```python
from build123d import *

# Parameters (mm, degrees)
SKETCH_2_W          = 100
SKETCH_2_H          = 70
EXTRUDE_1_DEPTH     = 80
SKETCH_4_W          = 96
SKETCH_4_H          = 66
CUT_EXTRUDE_1_DEPTH = 78
FILLET_2_R          = 2.5
SKETCH_6_R          = 5
SKETCH_6_R_2        = 2.3
EXTRUDE_3_DEPTH     = 10


with BuildPart() as part:
    # Эскиз2 → Бобышка-Вытянуть1 (new body)
    with BuildSketch(Plane(origin=(0, 0, 0), x_dir=(1, 0, 0), z_dir=(0, 1, 0))):
        Rectangle(SKETCH_2_W, SKETCH_2_H)
    extrude(amount=EXTRUDE_1_DEPTH)

    # Эскиз4 → Вырез-Вытянуть1 (cut)
    with BuildSketch(Plane(origin=(0, 80, 0), x_dir=(1, 0, 0), z_dir=(0, 1, 0))):
        Rectangle(SKETCH_4_W, SKETCH_4_H)
    extrude(amount=-CUT_EXTRUDE_1_DEPTH, mode=Mode.SUBTRACT)

    # Скругление2
    fillet_2_edges = [part.edges().sort_by_distance(p)[0] for p in [
        (-48, 2, 0),
        (-48, 41, 33),
        (0, 2, -33),
        (-48, 41, -33),
        (48, 2, 0),
        (48, 41, -33),
        (0, 2, 33),
        (48, 41, 33),
        (0, 0, 35),
        (-50, 0, 0),
        (0, 0, -35),
        (50, 0, 0),
        (50, 40, 35),
        (-50, 40, 35),
        (-50, 40, -35),
        (50, 40, -35),
    ]]
    fillet(fillet_2_edges, radius=FILLET_2_R)

    # Эскиз6 → Бобышка-Вытянуть3 (add)
    # profile 1 of 4: a face of its own
    with BuildSketch(Plane(origin=(0, 2, 0), x_dir=(1, 0, 0), z_dir=(0, 1, 0))):
        with Locations(Location((-37.5, 13.725, 0), (0, 0, 270))):
            Circle(SKETCH_6_R)
        with Locations(Location((-37.5, 13.725, 0), (0, 0, 270))):
            Circle(SKETCH_6_R_2, mode=Mode.SUBTRACT)
    # profile 2 of 4: a face of its own
    with BuildSketch(Plane(origin=(0, 2, 0), x_dir=(1, 0, 0), z_dir=(0, 1, 0))):
        with Locations(Location((37.5, 13.725, 0), (0, 0, 270))):
            Circle(SKETCH_6_R)
        with Locations(Location((37.5, 13.725, 0), (0, 0, 270))):
            Circle(SKETCH_6_R_2, mode=Mode.SUBTRACT)
    # profile 3 of 4: a face of its own
    with BuildSketch(Plane(origin=(0, 2, 0), x_dir=(1, 0, 0), z_dir=(0, 1, 0))):
        with Locations(Location((-37.5, -13.725, 0), (0, 0, 270))):
            Circle(SKETCH_6_R)
        with Locations(Location((-37.5, -13.725, 0), (0, 0, 270))):
            Circle(SKETCH_6_R_2, mode=Mode.SUBTRACT)
    # profile 4 of 4: a face of its own
    with BuildSketch(Plane(origin=(0, 2, 0), x_dir=(1, 0, 0), z_dir=(0, 1, 0))):
        with Locations(Location((37.5, -13.725, 0), (0, 0, 270))):
            Circle(SKETCH_6_R)
        with Locations(Location((37.5, -13.725, 0), (0, 0, 270))):
            Circle(SKETCH_6_R_2, mode=Mode.SUBTRACT)
    extrude(amount=EXTRUDE_3_DEPTH)


solid = part.part
```
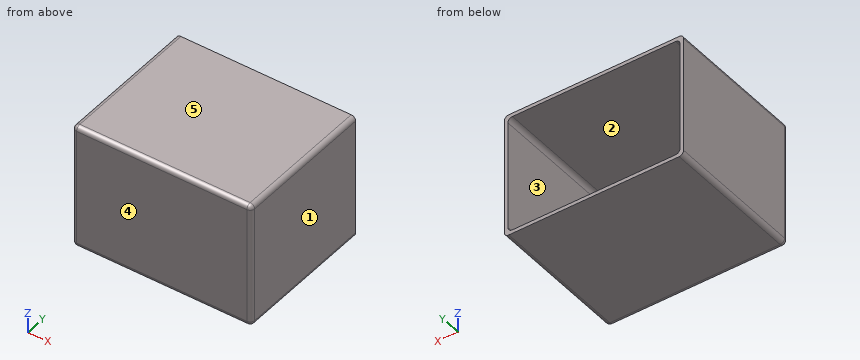
The model under review builds one solid part; all positions refer to its coordinate system, in mm. Face numbers are marked on the shaded views. A direction names the side the tool comes from. Round coordinates to 2 decimals unless told otherwise and drop trailing zeros. Write each loop counter-clockwise with the first axis right and the second up, starting at its lowest first coordinate (ties: lowest second). Pieces come first, ordered by that corner, then holes. Notation, with made-up numbers: (33, 25) -> (71, 25) arc R19 cw to (71, 52) -> close; hole circle Ø4 at (74, 10.25). An arc over 180 degrees is marked (long way). Use CSV: the item, a comma, the result in double quotes.
Q1. For the marked faces 1 and 2, list the 3-axis set-ups (+Z, -Z, +X, -X, +Y, -Y) from which the entire face can be reached by the end or side of a thin tool; tool diameter is ignored.
Checks:
face 1,"+Z, -Z, +X, +Y, -Y"
face 2,"+Y"
Q2. To check wall thickness, follow probe 1 along X at (y, z) = (10, -14); probe 2 along Z at (x, y) = (5.5, 42.5); probe 3 along X at (y, z) = (52.5, 1.5). State the ranges of each line that lie inside material, in increasing order. Write a range as [from, to].
Checks:
probe 1,"[-50, -48], [-42.49, -39.78], [-35.22, -32.51], [32.51, 35.22], [39.78, 42.49], [48, 50]"
probe 2,"[-35, -33], [33, 35]"
probe 3,"[-50, -48], [48, 50]"
Q3. Mouldability with a two-part tool opening along Z and no side actions: class the marked faces 3, 4 and 5 as released by +Z, released by -Z, zero draft, split by the parting line, or undercut.
Checks:
face 3,"undercut"
face 4,"zero draft"
face 5,"released by +Z"
Q4. Consider section C-C (z = 4). Give the boundary of the cut face in (x, y), then the cut area to 3 significant figures.
Checks:
outline,"(-50, 2.5) arc R2.5 ccw to (-47.5, 0) -> (47.5, 0) arc R2.5 ccw to (50, 2.5) -> (50, 80) -> (48, 80) -> (48, 4.5) arc R2.5 cw to (45.5, 2) -> (-45.5, 2) arc R2.5 cw to (-48, 4.5) -> (-48, 80) -> (-50, 80) -> close"
area,"512 mm²"
Q5. For pin 1 Ø3 at (x, z) = (-37.5, -13.725) entering from +Y; pin 2 Ø5 at (x, z) = (-37, 13.5) entering from +Y, all flat-tipped, find the tip position at first contact; note any pin that passes through.
Checks:
pin 1,"y = 2"
pin 2,"y = 12"
Q6. Consider section D-D (x = -37.5). Give the boundary of the cut face in (y, z) (3 decimals), then the cut area to 3 significant figures.
Checks:
outline,"(0, -32.5) arc R2.5 ccw to (2.5, -35) -> (80, -35) -> (80, -33) -> (4.5, -33) arc R2.5 cw to (2, -30.5) -> (2, -18.725) -> (12, -18.725) -> (12, -16.025) -> (2, -16.025) -> (2, -11.425) -> (12, -11.425) -> (12, -8.725) -> (2, -8.725) -> (2, 8.725) -> (12, 8.725) -> (12, 11.425) -> (2, 11.425) -> (2, 16.025) -> (12, 16.025) -> (12, 18.725) -> (2, 18.725) -> (2, 30.5) arc R2.5 cw to (4.5, 33) -> (80, 33) -> (80, 35) -> (2.5, 35) arc R2.5 ccw to (0, 32.5) -> close"
area,"560 mm²"
Q7. Consider section A-A (y = 73). Give the boundary of the cut face in (x, z).
Checks:
outline,"(-50, -32.5) arc R2.5 ccw to (-47.5, -35) -> (47.5, -35) arc R2.5 ccw to (50, -32.5) -> (50, 32.5) arc R2.5 ccw to (47.5, 35) -> (-47.5, 35) arc R2.5 ccw to (-50, 32.5) -> close; hole (-48, -30.5) arc R2.5 ccw to (-45.5, -33) -> (45.5, -33) arc R2.5 ccw to (48, -30.5) -> (48, 30.5) arc R2.5 ccw to (45.5, 33) -> (-45.5, 33) arc R2.5 ccw to (-48, 30.5) -> close"
Q8. Consider section B-B (x = -16.5). Give the boundary of the cut face in (y, z).
Checks:
outline,"(0, -32.5) arc R2.5 ccw to (2.5, -35) -> (80, -35) -> (80, -33) -> (4.5, -33) arc R2.5 cw to (2, -30.5) -> (2, 30.5) arc R2.5 cw to (4.5, 33) -> (80, 33) -> (80, 35) -> (2.5, 35) arc R2.5 ccw to (0, 32.5) -> close"
